Build history of the part. All positions in model axes, mm. Round coordinates to 2 decimals unless told otherwise and drop trailing zeros. Write each loop counter-clockwise with the first axis right and the second up, starting at its lowest first coordinate (ties: lowest second). Pieces come first, ordered by that corner, then holes.
Item 1: Wall check: probe 1 along X at (y, z) = (30, -7.5); probe 2 along Y at (x, z) = (-37.5, -11.5); probe 3 along X at (y, z) = (-27.5, -4.5). Give the ranges that are in metal, low to high.
Item 2: Band-saw the part on D-D, the plane x = -7.5. Write the cut outline in (y, z), then the cut area to 3 significant figures.
Item 3: Band-saw the part on C-C, the plane y = 30. Write the cut outline in (x, z), then the cut area to 3 significant figures.
Item 4: Band-saw the part on B-B, the plane x = 27.5. Write the cut outline in (y, z), then the cut area to 3 significant figures.
Item 5: Drop flat-ended pins along their axis: pin 1 Ø3.5 at (x, y) = (-37.5, 30) entering from +Z; pin 2 Ø8 at (x, y) = (-37.5, -30) entering from +Z; pin 3 Ø10 at (x, y) = (10, -12) entering from +Z; pin 4 Ø7 at (x, y) = (-7.5, 30) entering from +Z. Give the stop position or say it passes through.
Item 6: Band-saw the part on A-A, the plane y = -40. Write the cut outline in (x, z).
```python
from build123d import *

# Parameters (mm, degrees)
F0_W           = 95
F0_H           = 120
F0_R           = 3
F1_DEPTH       = 15
F2_D           = 6
F2_CSINK_D     = 12
F2_CSINK_ANGLE = 90
F3_D           = 6


with BuildPart() as f1:
    # F0 (on Top) → F1 (new body)
    with BuildSketch(Plane.XY):
        Rectangle(F0_W, F0_H)
        with Locations((-37.5, -30)):
            Circle(F0_R, mode=Mode.SUBTRACT)
        with Locations((-7.5, -30)):
            Circle(F0_R, mode=Mode.SUBTRACT)
        with Locations((27.5, -40)):
            Circle(F0_R, mode=Mode.SUBTRACT)
        with Locations((-37.5, 30)):
            Circle(F0_R, mode=Mode.SUBTRACT)
        with Locations((-7.5, 30)):
            Circle(F0_R, mode=Mode.SUBTRACT)
        with Locations((27.5, 40)):
            Circle(F0_R, mode=Mode.SUBTRACT)
        with Locations((-37.5, 30)):
            Circle(F0_R)
        with Locations((-37.5, -30)):
            Circle(F0_R)
        with Locations((-7.5, -30)):
            Circle(F0_R)
        with Locations((27.5, -40)):
            Circle(F0_R)
        with Locations((-7.5, 30)):
            Circle(F0_R)
        with Locations((27.5, 40)):
            Circle(F0_R)
    extrude(amount=-F1_DEPTH)

    # F2 (through all)
    with Locations(Plane.XY):
        with Locations((-37.5, 30), (-7.5, 30), (-37.5, -30), (-7.5, -30)):
            CounterSinkHole(F2_D / 2, F2_CSINK_D / 2, counter_sink_angle=F2_CSINK_ANGLE)

    # F3 (through all)
    with Locations(Plane.XY):
        with Locations((27.5, 40), (27.5, -40)):
            Hole(F3_D / 2)


solid = f1.part
```
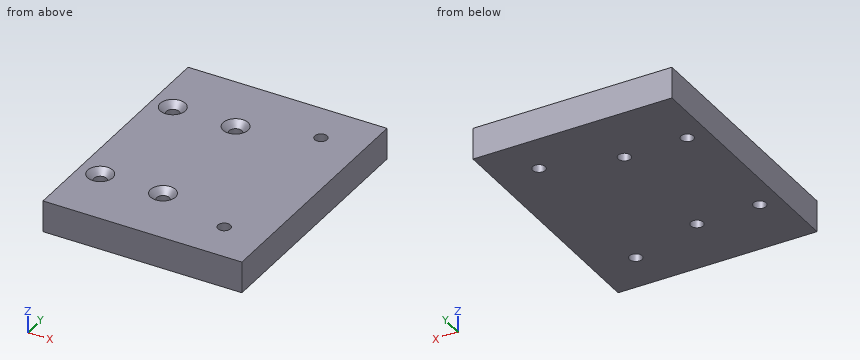
Results:
1. probe 1: x = -47.5 to -40.5, -34.5 to -10.5, -4.5 to 47.5
1. probe 2: y = -60 to -33, -27 to 27, 33 to 60
1. probe 3: x = -47.5 to -39.16, -35.84 to -9.16, -5.84 to 47.5
2. outline: (-60, -15) - (-33, -15) - (-33, -3) - (-36, 0) - (-60, 0) - close; (-27, -15) - (27, -15) - (27, -3) - (24, 0) - (-24, 0) - (-27, -3) - close; (33, -15) - (60, -15) - (60, 0) - (36, 0) - (33, -3) - close
2. area: 1,600 mm2
3. outline: (-47.5, -15) - (-40.5, -15) - (-40.5, -3) - (-43.5, 0) - (-47.5, 0) - close; (-34.5, -15) - (-10.5, -15) - (-10.5, -3) - (-13.5, 0) - (-31.5, 0) - (-34.5, -3) - close; (-4.5, -15) - (47.5, -15) - (47.5, 0) - (-1.5, 0) - (-4.5, -3) - close
3. area: 1,230 mm2
4. outline: (-60, -15) - (-43, -15) - (-43, 0) - (-60, 0) - close; (-37, -15) - (37, -15) - (37, 0) - (-37, 0) - close; (43, -15) - (60, -15) - (60, 0) - (43, 0) - close
4. area: 1,620 mm2
5. pin 1: passes through
5. pin 2: stops at z = -2
5. pin 3: stops at z = 0
5. pin 4: stops at z = -2.5
6. outline: (-47.5, -15) - (24.5, -15) - (24.5, 0) - (-47.5, 0) - close; (30.5, -15) - (47.5, -15) - (47.5, 0) - (30.5, 0) - close
